Drawing for the job (mm, zero at the part's lowest x, y, z). A direction names the side the tool comes from. Coordinates: 2 decimals unless noted, no trailing zeros. Write each loop counter-clockwise with the first axis right and the second up, starting at its lowest first coordinate (ties: lowest second). Pieces come first, ordered by that corner, then holes. Notation, with made-up numbers: M 1.5,32 L 30.5,32 A14 cw 30.5,40 Z; hole C 79.5,51 d11. An arc over 180 degrees is marked long. Use a Markdown table: item, result. Add a question column.
Q1. Slice it at A-A on x = 142. Write the cut outline in (y, z), then the cut area to 3 significant figures.
Q2. Mould opens along X. For the marked faces 1, 2 and 3 say: released by +X, released by -X, zero draft, split by the parting line, or undercut.
Q3. Tool access for the marked faces 4, 5 and 6: list every direction of +Z, -Z, +X, -X, +Y, -Y with a clear straight run to the whole face (end or side of a thin tool).
Q4. Slice it at D-D on z = 75. Write the cut outline in (x, y), then the cut area to 3 significant figures.
Q5. Wall check: L1, parallel to X at y = 4, z = 57; L2, parallel to Z at x = 20, y = 4; L3, parallel to X at y = 6.75, z = 68. Give the ranges that are in metal, low to high. Write a range as from..to.
Q6. Slice it at C-C on z = 59. Write the cut outline in (x, y).
Q7. Slice it at B-B on y = 4.75. Write the cut outline in (x, z).
Q8. Pin check, flat tips, straight feed: pin 1 Ø2.5 at (y, z) = (2, 51) entering from -X; pin 2 Ø1.5 at (y, z) = (11.5, 39.5) entering from +X; pin 3 Ø2 at (x, z) = (127.5, 32.5) entering from +Y; pin 4 Ø9 at (x, z) = (142, 68) entering from -Y. Stop position of each tip, or through.
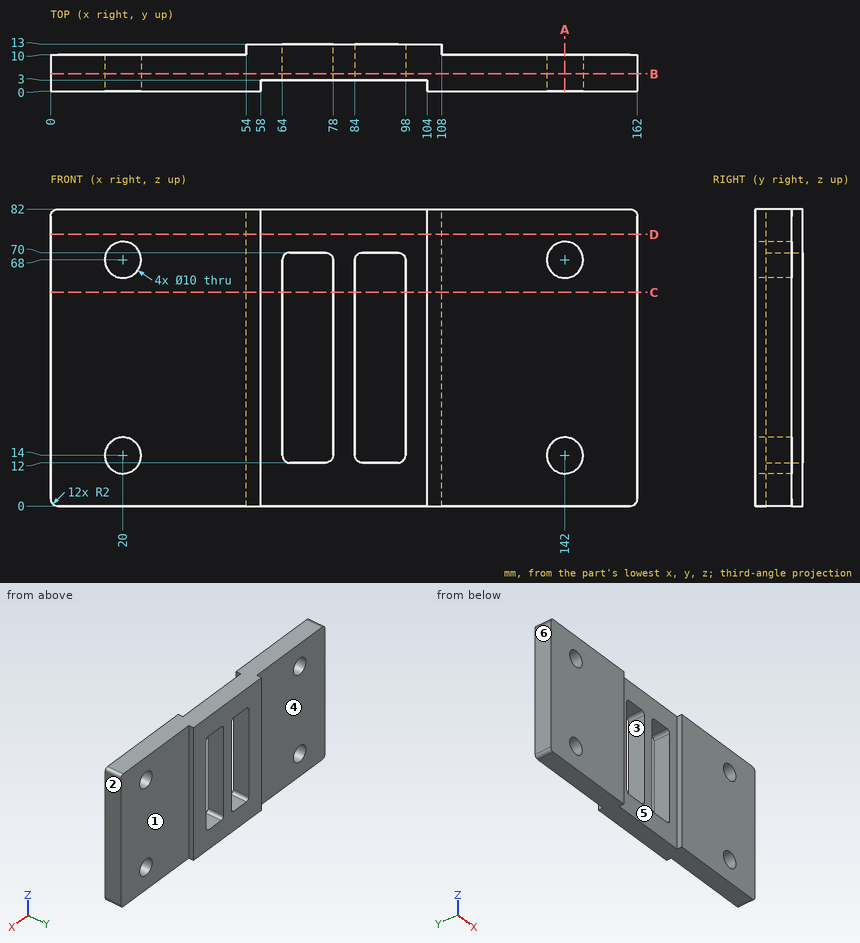
Recorded:
| question | item | result |
|---|---|---|
| 1 | outline | M 0,0 L 10,0 L 10,9 L 0,9 Z; M 0,19 L 10,19 L 10,63 L 0,63 Z; M 0,73 L 10,73 L 10,82 L 0,82 Z |
| 1 | area | 620 mm² |
| 2 | face 1 | zero draft |
| 2 | face 2 | released by +X |
| 2 | face 3 | undercut |
| 3 | face 4 | +Z, -Z, -X, +Y |
| 3 | face 5 | +Z, -Z, -Y |
| 3 | face 6 | +Z, -Z, -X, +Y, -Y |
| 4 | outline | M 0,0 L 58,0 L 58,3 L 104,3 L 104,0 L 162,0 L 162,10 L 108,10 L 108,13 L 54,13 L 54,10 L 0,10 Z |
| 4 | area | 1,640 mm² |
| 5 | L1 | 0..64, 78..84, 98..162 |
| 5 | L2 | 0..9, 19..63, 73..82 |
| 5 | L3 | 0..15, 25..64, 78..84, 98..137, 147..162 |
| 6 | outline | M 0,0 L 58,0 L 58,3 L 64,3 L 64,13 L 54,13 L 54,10 L 0,10 Z; M 78,3 L 84,3 L 84,13 L 78,13 Z; M 98,3 L 104,3 L 104,0 L 162,0 L 162,10 L 108,10 L 108,13 L 98,13 Z |
| 7 | outline | M 0,2 A2 ccw 2,0 L 160,0 A2 ccw 162,2 L 162,80 A2 ccw 160,82 L 2,82 A2 ccw 0,80 Z; hole C 20,14 d10; hole C 20,68 d10; hole M 64,14 A2 ccw 66,12 L 76,12 A2 ccw 78,14 L 78,68 A2 ccw 76,70 L 66,70 A2 ccw 64,68 Z; hole M 84,14 A2 ccw 86,12 L 96,12 A2 ccw 98,14 L 98,68 A2 ccw 96,70 L 86,70 A2 ccw 84,68 Z; hole C 142,14 d10; hole C 142,68 d10 |
| 8 | pin 1 | x = 0 |
| 8 | pin 2 | x = 108 |
| 8 | pin 3 | y = 10 |
| 8 | pin 4 | through |
